```python
from build123d import *

# Parameters (mm, degrees)
SKETCH2_W           = 23.876
SKETCH2_H           = 35.052
SKETCH2_R           = 1.143
SKETCH2_R_2         = 0.635
BOSS_EXTRUDE1_DEPTH = 3.175
SKETCH3_W           = 6.35
SKETCH3_H           = 35.052
BOSS_EXTRUDE2_DEPTH = 6.35
SKETCH4_R           = 1.143
CUT_EXTRUDE3_DEPTH  = 49.53
SKETCH5_W           = 6.35
SKETCH5_H           = 9.652
CUT_EXTRUDE4_DEPTH  = 24.765
CUT_EXTRUDE5_DEPTH  = 49.53


with BuildPart() as part:
    # Sketch2 → Boss-Extrude1 (new body)
    with BuildSketch(Plane.XY):
        with Locations((0, 17.526)):
            Rectangle(SKETCH2_W, SKETCH2_H)
        with Locations((-5.08, 11.938)):
            Circle(SKETCH2_R, mode=Mode.SUBTRACT)
        with Locations((5.08, 11.938)):
            Circle(SKETCH2_R, mode=Mode.SUBTRACT)
        with Locations((-8.128, 17.526)):
            Circle(SKETCH2_R_2, mode=Mode.SUBTRACT)
        with Locations((8.128, 17.526)):
            Circle(SKETCH2_R_2, mode=Mode.SUBTRACT)
    extrude(amount=BOSS_EXTRUDE1_DEPTH)

    # Sketch3 → Boss-Extrude2 (add)
    with BuildSketch(Plane.XY.offset(3.175)):
        with Locations((0, 17.526)):
            Rectangle(SKETCH3_W, SKETCH3_H)
    extrude(amount=BOSS_EXTRUDE2_DEPTH)

    # Sketch4 → Cut-Extrude3 (cut)
    with BuildSketch(Plane(origin=(0, 0, 0), x_dir=(1, 0, 0), z_dir=(0, 1, 0))):
        with Locations((0, -6.35)):
            Circle(SKETCH4_R)
    extrude(amount=CUT_EXTRUDE3_DEPTH, mode=Mode.SUBTRACT)

    # Sketch5 → Cut-Extrude4 (cut, symmetric)
    with BuildSketch(Plane(origin=(0, 0, 0), x_dir=(0, 0, -1), z_dir=(1, 0, 0))):
        with Locations((-6.35, 17.526)):
            Rectangle(SKETCH5_W, SKETCH5_H)
    extrude(amount=CUT_EXTRUDE4_DEPTH, both=True, mode=Mode.SUBTRACT)

    # Sketch6 → Cut-Extrude5 (cut)
    with BuildSketch(Plane(origin=(0, 0, 0), x_dir=(1, 0, 0), z_dir=(0, 1, 0))):
        with BuildLine():
            ThreePointArc((0, -9.525), (-2.24506403, -8.59506403), (-3.175, -6.35))
            Line((-3.175, -6.35), (-3.175, -9.525))
            Line((-3.175, -9.525), (0, -9.525))
        make_face()
        with BuildLine():
            ThreePointArc((3.175, -6.35), (2.24506403, -8.59506403), (0, -9.525))
            Line((0, -9.525), (3.175, -9.525))
            Line((3.175, -9.525), (3.175, -6.35))
        make_face()
    extrude(amount=CUT_EXTRUDE5_DEPTH, mode=Mode.SUBTRACT)


solid = part.part
```
CAD build for the part. Positions are in the model's coordinates, mm. A direction names the side the tool comes from. Round coordinates to 2 decimals unless told otherwise and drop trailing zeros. Write each loop counter-clockwise with the first axis right and the second up, starting at its lowest first coordinate (ties: lowest second). Pieces come first, ordered by that corner, then holes. Notation, with made-up numbers: M 69.25,-5.5 L 127.25,-5.5 A33 cw 127.25,23.5 Z; hole C -33,-21.5 d7. An arc over 180 degrees is marked long. One line per question, with ' | ' between items.
1. Which spindle directions (+Z, -Z, +X, -X, +Y, -Y) get a long thin tool onto all of the face, cutting with end or side? Do faces 1 (the cylindrical face through (-4.024, 11.5, 1.565)), 2 (the flat face through (-3.175, 6, 5)), 3 (the flat face through (0, 12.7, 5)), 4 (the flat face through (3.175, 29, 5)). Say none if no direction does.
Working result:
face 1: +Z, -Z | face 2: +Z, -X, +Y, -Y | face 3: +Z, +X, -X | face 4: +Z, +X, +Y, -Y
2. Cut at C-C on y = 29.5. Write the cut outline in (x, z) (3 decimals), and give its area (3 significant figures).
Working result:
outline: M -11.938,0 L 11.938,0 L 11.938,3.175 L 3.175,3.175 L 3.175,6.35 A3.175 ccw -3.175,6.35 L -3.175,3.175 L -11.938,3.175 Z; hole C 0,6.35 d2.286 | area: 108 mm2
3. Cut at B-B on z = 4.5. Write the cut outline in (x, y) (3 decimals).
Working result:
outline: M -3.175,0 L 3.175,0 L 3.175,12.7 L -3.175,12.7 Z; M -3.175,22.352 L 3.175,22.352 L 3.175,35.052 L -3.175,35.052 Z
4. Mould opens along Z. For faces 5 (the cylindrical face through (-0.248, 28.613, 7.466)), 6 (the flat face through (11.938, 17, 2)), 7 (the flat face through (0, 18, 0)), 8 (the cylindrical face through (-0.248, 6.261, 7.466)) say: pulls with the +Z half, pulls with the -Z half, needs draft (parallel to the pull), parting line crosses it, or undercut.
Working result:
face 5: undercut | face 6: needs draft | face 7: pulls with the -Z half | face 8: undercut
5. Cut at D-D on x = 0.5. Write the cut outline in (y, z) (3 decimals), and give its area (3 significant figures).
Working result:
outline: M 0,0 L 35.052,0 L 35.052,5.322 L 22.352,5.322 L 22.352,3.175 L 12.7,3.175 L 12.7,5.322 L 0,5.322 Z; M 0,7.378 L 12.7,7.378 L 12.7,9.485 L 0,9.485 Z; M 22.352,7.378 L 35.052,7.378 L 35.052,9.485 L 22.352,9.485 Z | area: 219 mm2
6. Cut at A-A on x = 5.08. Write the cut outline in (y, z) (3 decimals).
Working result:
outline: M 0,0 L 10.795,0 L 10.795,3.175 L 0,3.175 Z; M 13.081,0 L 35.052,0 L 35.052,3.175 L 13.081,3.175 Z
7. Probe L1, parallel to Y at x = 5.08, z = 2.4 (3 decimals); L2, parallel to X at y = 11.5, z = 3; L3, parallel to X at y = 4.5, z = 6.35 (3 decimals). List the from-to ranges inside material, lowest first. Write a range as from..to.
Working result:
L1: 0..10.795, 13.081..35.052 | L2: -11.94..-6.14, -4.02..4.02, 6.14..11.94 | L3: -3.175..-1.143, 1.143..3.175
8. Pin check, flat tips, straight feed: pin 1 Ø2.5 at (x, y) = (-5.08, 11.938) entering from +Z (3 decimals); pin 2 Ø2.5 at (y, z) = (4.5, 4.5) entering from -X (3 decimals). Stop position of each tip, or through.
Working result:
pin 1: z = 3.175 | pin 2: x = -3.175
